```python
from build123d import *

# Parameters (mm, degrees)
SKETCH1_W           = 25.4
SKETCH1_H           = 49.53
BOSS_EXTRUDE2_DEPTH = 12.7
SKETCH2_W           = 8.89
SKETCH2_H           = 21.59
SKETCH2_W_2         = 11.324200872
SKETCH2_H_2         = 7.724794812
SKETCH2_H_3         = 7.62
CUT_EXTRUDE1_DEPTH  = 6.35


with BuildPart() as part:
    # Sketch1 → Boss-Extrude2 (new body)
    with BuildSketch(Plane.XY):
        with Locations((-15.1641049, 1.570131369)):
            Rectangle(SKETCH1_W, SKETCH1_H)
    extrude(amount=BOSS_EXTRUDE2_DEPTH)

    # Sketch2 → Cut-Extrude1 (cut)
    with BuildSketch(Plane.XY.offset(12.7)):
        with Locations((-23.4191049, -9.859868631)):
            Rectangle(SKETCH2_W, SKETCH2_H)
        with Locations((-10.772004464, -15.522471225)):
            Rectangle(SKETCH2_W_2, SKETCH2_H_2)
        with Locations((-9.4491049, -4.040073819)):
            Rectangle(SKETCH2_W, SKETCH2_H_3)
        with Locations((-23.066267196, 8.555131369)):
            Rectangle(SKETCH2_W, SKETCH2_H_3)
        with Locations((-11.636267196, 7.389926181)):
            Rectangle(SKETCH2_W, SKETCH2_H_3)
        with Locations((-23.066267196, 19.985131369)):
            Rectangle(SKETCH2_W, SKETCH2_H_3)
        with Locations((-11.636267196, 18.819926181)):
            Rectangle(SKETCH2_W, SKETCH2_H_3)
    extrude(amount=-CUT_EXTRUDE1_DEPTH, mode=Mode.SUBTRACT)


solid = part.part
```
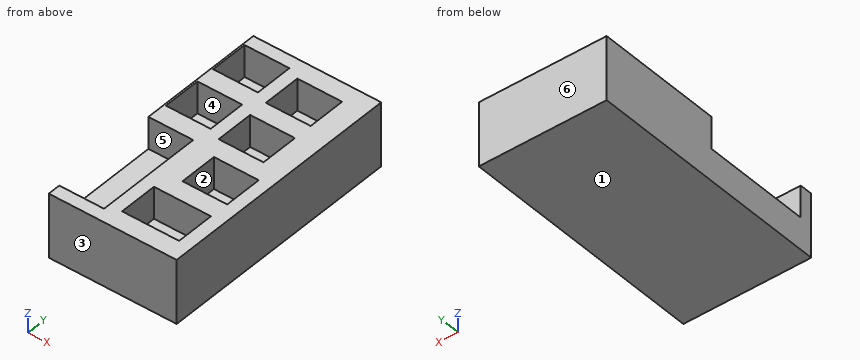
Input: part model. Units: mm. Frame: model coordinates. Face numbers are marked on the shaded views. A direction names the side the tool comes from. Coordinates: 2 decimals unless noted, no trailing zeros. Write each loop counter-clockwise with the first axis right and the second up, starting at its lowest first coordinate (ties: lowest second). Pieces come first, ordered by that corner, then holes. Notation, with made-up numbers: (2, 33) - (22, 33) arc R20 cw to (22, 50) - close; hole circle Ø2 at (37, 13). An arc over 180 degrees is marked (long way). Put each result on its own line as item: value. Start each with the question number.
1) Cut plane B-B (z = 8.5). State how many separate pieces and enclosed holes the cut face has, plus the area to 3 significant figures.
2) Cut plane C-C (y = 9). Return the cut outline in (x, z).
3) Cut plane D-D (y = -18). Return the cut outline in (x, z).
4) Mould query, pull axis Y, two halves, no side actions, for the marked faces 1, 2 and 3. Classes: pulls with the +Y half, pulls with the -Y half, needs draft (parallel to the pull), parting line crosses it, or undercut.
5) Contact query for flat-ended pins moving along their axis: pin 1 (4 mm diameter, centred on x = -7, y = -13.5, fed in from -Z); pin 2 (2.5 mm diameter, centred on x = -7.5, y = -4.5, fed in from +Z); pin 3 (5 mm diameter, centred on y = -4.5, z = 9, fed in from -X). Output: stop coordinate, or through.
6) Cut plane A-A (x = -23). Return the cut outline in (y, z).
7) Ray query, L1, parallel to Y at x = -10.75, z = 10.5; L2, parallel to Y at x = -15.75, z = 10.5; L3, parallel to X at y = -7, z = 12. Return the intervals inside material, ascending.
8) Reachability of the marked faces 4, 5 and 6 from +Z, -Z, +X, -X, +Y, -Y: full face, straight path, thin tool, end or side. Return the list, or none.
Resolved:
1. separate pieces: 1
1. enclosed holes: 6
1. area: 640 mm2
2. outline: (-27.86, 0) - (-2.46, 0) - (-2.46, 12.7) - (-7.19, 12.7) - (-7.19, 6.35) - (-16.08, 6.35) - (-16.08, 12.7) - (-18.62, 12.7) - (-18.62, 6.35) - (-27.51, 6.35) - (-27.51, 12.7) - (-27.86, 12.7) - close
3. outline: (-27.86, 0) - (-2.46, 0) - (-2.46, 12.7) - (-5.11, 12.7) - (-5.11, 6.35) - (-16.43, 6.35) - (-16.43, 12.7) - (-18.97, 12.7) - (-18.97, 6.35) - (-27.86, 6.35) - close
4. face 1: needs draft
4. face 2: undercut
4. face 3: pulls with the -Y half
5. pin 1: stops at z = 0
5. pin 2: stops at z = 6.35
5. pin 3: stops at x = -18.97
6. outline: (-23.19, 0) - (26.34, 0) - (26.34, 12.7) - (23.8, 12.7) - (23.8, 6.35) - (16.18, 6.35) - (16.18, 12.7) - (12.37, 12.7) - (12.37, 6.35) - (4.75, 6.35) - (4.75, 12.7) - (0.94, 12.7) - (0.94, 6.35) - (-20.65, 6.35) - (-20.65, 12.7) - (-23.19, 12.7) - close
7. L1: y = -23.19 to -19.38, -11.66 to -7.85, -0.23 to 3.58, 11.2 to 15.01, 22.63 to 26.34
7. L2: y = -23.19 to -19.38, -11.66 to 3.58, 11.2 to 15.01, 22.63 to 26.34
7. L3: x = -18.97 to -13.89, -5 to -2.46
8. face 4: +Z
8. face 5: +Z, -X
8. face 6: +Z, -Z, +X, -X, +Y
